Input: part model. Units: mm. Frame: model coordinates. A direction names the side the tool comes from. Coordinates: 2 decimals unless noted, no trailing zeros. Write each loop counter-clockwise with the first axis right and the second up, starting at its lowest first coordinate (ties: lowest second). Pieces come first, ordered by that corner, then holes. Notation, with made-up numbers: (-34.5, 42) -> (-27.5, 42) arc R29 ccw to (-27.5, 78) -> close; hole circle Ø3 at (54, -27.75). An arc over 180 degrees is marked (long way). One line per question, with ' | ' between items. Start each with the question number.
```python
from build123d import *

# Parameters (mm, degrees)
SKETCH15_R            = 5
BOSS_EXTRUDE7_DEPTH   = 21.5
CUT_EXTRUDE6_DEPTH    = 52.132181647
CUT_EXTRUDE7_DEPTH    = 52.132181647
M3_TAPPED_HOLE1_D     = 2.5
M3_TAPPED_HOLE2_D     = 2.5
M3_TAPPED_HOLE2_DEPTH = 7.5
M3_TAPPED_HOLE2_TIP   = 0.751075774


with BuildPart() as part:
    # Sketch15 → Boss-Extrude7 (new, symmetric)
    with BuildSketch(Plane.XY):
        with BuildLine():
            Line((-9.526279442, 70), (9.526279442, 70))
            ThreePointArc((9.526279442, 70), (11.356406461, 71.830127019), (13.856406461, 72.5))
            Line((13.856406461, 72.5), (32.346493939, 72.5))
            ThreePointArc((32.346493939, 72.5), (33.794607035, 72.872649917), (34.882960648, 73.898021026))
            Line((34.882960648, 73.898021026), (39.536466709, 81.266072289))
            ThreePointArc((39.536466709, 81.266072289), (39.881787651, 82.034204793), (40, 82.868051264))
            Line((40, 82.868051264), (40, 93.5))
            Line((40, 93.5), (34, 93.5))
            Line((34, 93.5), (34, 82.868051264))
            ThreePointArc((34, 82.868051264), (33.881787651, 82.034204793), (33.536466709, 81.266072289))
            Line((33.536466709, 81.266072289), (32.672434332, 79.898021026))
            ThreePointArc((32.672434332, 79.898021026), (31.584080719, 78.872649917), (30.135967623, 78.5))
            Line((30.135967623, 78.5), (13.856406461, 78.5))
            ThreePointArc((13.856406461, 78.5), (11.356406461, 79.169872981), (9.526279442, 81))
            Line((9.526279442, 81), (-9.526279442, 81))
            ThreePointArc((-9.526279442, 81), (-11.356406461, 79.169872981), (-13.856406461, 78.5))
            Line((-13.856406461, 78.5), (-30.135967623, 78.5))
            ThreePointArc((-30.135967623, 78.5), (-31.584080719, 78.872649917), (-32.672434332, 79.898021026))
            Line((-32.672434332, 79.898021026), (-33.536466709, 81.266072289))
            ThreePointArc((-33.536466709, 81.266072289), (-33.881787651, 82.034204793), (-34, 82.868051264))
            Line((-34, 82.868051264), (-34, 93.5))
            Line((-34, 93.5), (-40, 93.5))
            Line((-40, 93.5), (-40, 82.868051264))
            ThreePointArc((-40, 82.868051264), (-39.881787651, 82.034204793), (-39.536466709, 81.266072289))
            Line((-39.536466709, 81.266072289), (-34.882960648, 73.898021026))
            ThreePointArc((-34.882960648, 73.898021026), (-33.794607035, 72.872649917), (-32.346493939, 72.5))
            Line((-32.346493939, 72.5), (-13.856406461, 72.5))
            ThreePointArc((-13.856406461, 72.5), (-11.356406461, 71.830127019), (-9.526279442, 70))
        make_face()
        with Locations((0, 75.5)):
            Circle(SKETCH15_R, mode=Mode.SUBTRACT)
    extrude(amount=BOSS_EXTRUDE7_DEPTH, both=True)

    # Sketch16 → Cut-Extrude6 (cut, through all)
    with BuildSketch(Plane.XZ.offset(-70)):
        Polygon((-9.526279442, 3.5), (-13.856406461, 3.5), (-34, 21.5), (34, 21.5), (13.856406461, 3.5), (9.526279442, 3.5), align=None)
        Polygon((-9.526279442, -7.5), (-13.856406461, -7.5), (-34, -21.5), (34, -21.5), (13.856406461, -7.5), (9.526279442, -7.5), align=None)
    extrude(amount=-CUT_EXTRUDE6_DEPTH, mode=Mode.SUBTRACT)

    # Sketch18 → Cut-Extrude7 (cut, through all)
    with BuildSketch(Plane.XZ.offset(-70)):
        with BuildLine():
            Line((-19.430135511, 0.434122818), (-30.959972352, 10.737004611))
            ThreePointArc((-30.959972352, 10.737004611), (-31.889114835, 11.302767724), (-32.95892467, 11.5))
            Line((-32.95892467, 11.5), (-40, 11.5))
            Line((-40, 11.5), (-40, -11.5))
            Line((-40, -11.5), (-31.065089761, -11.5))
            ThreePointArc((-31.065089761, -11.5), (-30.167975157, -11.362723421), (-29.352962435, -10.963456925))
            Line((-29.352962435, -10.963456925), (-19.716960503, -4.266338718))
            ThreePointArc((-19.716960503, -4.266338718), (-18.434657551, -1.985603731), (-19.430135511, 0.434122818))
        make_face()
        with BuildLine():
            Line((40, -11.5), (31.065089761, -11.5))
            ThreePointArc((31.065089761, -11.5), (30.167975157, -11.362723421), (29.352962435, -10.963456925))
            Line((29.352962435, -10.963456925), (19.716960503, -4.266338718))
            ThreePointArc((19.716960503, -4.266338718), (18.434657551, -1.985603731), (19.430135511, 0.434122818))
            Line((19.430135511, 0.434122818), (30.959972352, 10.737004611))
            ThreePointArc((30.959972352, 10.737004611), (31.889114835, 11.302767724), (32.95892467, 11.5))
            Line((32.95892467, 11.5), (40, 11.5))
            Line((40, 11.5), (40, -11.5))
        make_face()
    extrude(amount=-CUT_EXTRUDE7_DEPTH, mode=Mode.SUBTRACT)

    # M3 Tapped Hole1 (through all)
    with Locations(Plane(origin=(-8, 75.5, 3.5), x_dir=(1, 0, 0), z_dir=(0, 0, 1))):
        with Locations((0, 0), (16, 0)):
            Hole(M3_TAPPED_HOLE1_D / 2)

    # M3 Tapped Hole2
    with Locations(Plane(origin=(-37, 93.5, -15.5), x_dir=(0, 0, 1), z_dir=(0, 1, 0))):
        with Locations((0, 0), (0, 74), (31, 74), (31, 0)):
            Hole(M3_TAPPED_HOLE2_D / 2, depth=M3_TAPPED_HOLE2_DEPTH)
            with Locations((0, 0, -(M3_TAPPED_HOLE2_DEPTH + M3_TAPPED_HOLE2_TIP / 2))):  # 118° drill point
                Cone(0, M3_TAPPED_HOLE2_D / 2, M3_TAPPED_HOLE2_TIP, mode=Mode.SUBTRACT)


solid = part.part
```
1) Section A-A, the plane y = 91.25. Return loops of the section in (x, z), then the cut area to 3 significant figures.
2) Ray query, line 1 (X direction, y = 75.5, z = -1.75); line 2 (X direction, y = 89.5, z = 15.5); line 3 (Z direction, x = 37, y = 91.5). Return the intervals inside material, ascending.
3) First-contact query: P1, Ø20.5, axis at x = 25.5, z = 3, coming from the -Y side; P2, Ø6, axis at x = 30, y = 90.5, coming from the +Z side; P3, Ø18, axis at x = -23, z = 2, coming from the +Y side; P4, Ø8, axis at y = 76, z = -1, coming from the +X side. Flat tips, straight axial feed; report the tip coordinate or a pass-through.
4) Pull-direction query (X, two-part tool) for faces 5 (the face through (-33.81, 72.88, 16.54)), 6 (the face through (24.07, 75.31, -14.6)), 7 (the face through (40, 88, -16)); classes: released by +X, released by -X, zero draft, split by the parting line, or undercut.
5) Access query for faces 1 (the face through (36, 83, -11.5)), 2 (the face through (-38.22, 89.7, 15.77)), 3 (the face through (31.6, 78.88, 15.23)), 4 (the face through (-3, 71, 3.5)). Directions: +Z, -Z, +X, -X, +Y, -Y. A direction counts if a zero-diameter tool reaches every point of the face in a straight line with its end or side. Return the directions, or none.
6) Section B-B, the plane x = 0. Return loops of the section in (y, z), then the cut area to 3 significant figures.
7) Section C-C, the plane z = 5. Return loops of the section in (x, y).
8) Section D-D, the plane y = 75.5. Give the number of separate pieces and of enclosed holes in the cut face, then the cut area to 3 significant figures.
Answer block:
1) outline: (-40, -21.5) -> (-34, -21.5) -> (-34, -11.5) -> (-40, -11.5) -> close; (-40, 11.5) -> (-34, 11.5) -> (-34, 21.5) -> (-40, 21.5) -> close; (34, -21.5) -> (40, -21.5) -> (40, -11.5) -> (34, -11.5) -> close; (34, 11.5) -> (40, 11.5) -> (40, 21.5) -> (34, 21.5) -> close; hole circle Ø2.5 at (-37, -15.5); hole circle Ø2.5 at (-37, 15.5); hole circle Ø2.5 at (37, -15.5); hole circle Ø2.5 at (37, 15.5) | area: 220 mm2
2) line 1: x = -18.43 to -9.25, -6.75 to -5, 5 to 6.75, 9.25 to 18.43 | line 2: x = -40 to -38.25, -35.75 to -34, 34 to 35.75, 38.25 to 40 | line 3: z = -21.5 to -16.75, -14.25 to -11.5, 11.5 to 14.25, 16.75 to 21.5
3) P1: stops at y = 72.5 | P2: passes through | P3: stops at y = 78.5 | P4: stops at x = 22.3
4) face 5: released by -X | face 6: undercut | face 7: released by +X
5) face 1: +X, +Y, -Y | face 2: +Y | face 3: +Z, -Z, +Y | face 4: +Z, +Y, -Y
6) outline: (70, -7.5) -> (70.5, -7.5) -> (70.5, 3.5) -> (70, 3.5) -> close; (80.5, -7.5) -> (81, -7.5) -> (81, 3.5) -> (80.5, 3.5) -> close | area: 11.0 mm2
7) outline: (-24.54, 72.5) -> (-15.54, 72.5) -> (-15.54, 78.5) -> (-24.54, 78.5) -> close; (15.54, 72.5) -> (24.54, 72.5) -> (24.54, 78.5) -> (15.54, 78.5) -> close
8) separate pieces: 4 | enclosed holes: 0 | area: 844 mm2
